from build123d import *

# Parameters (mm, degrees)
F0_W     = 100.4
F0_H     = 100.4
F0_W_2   = 87.7
F0_H_2   = 87.7
F1_DEPTH = 6.35
F2_DEPTH = 119.05


with BuildPart() as f1:
    # F0 (on Front) → F1 (new body)
    with BuildSketch(Plane.XZ):
        with Locations((0, 50.2)):
            Rectangle(F0_W, F0_H)
        with Locations((0, 50.2)):
            Rectangle(F0_W_2, F0_H_2, mode=Mode.SUBTRACT)
        with Locations((0, 50.2)):
            Rectangle(F0_W_2, F0_H_2)
    extrude(amount=F1_DEPTH)

    # F0 (on Front) → F2 (join)
    with BuildSketch(Plane.XZ):
        with Locations((0, 50.2)):
            Rectangle(F0_W, F0_H)
        with Locations((0, 50.2)):
            Rectangle(F0_W_2, F0_H_2, mode=Mode.SUBTRACT)
    extrude(amount=F2_DEPTH)


solid = f1.part
Verification items for the finished model (mm, model axes). A direction names the side the tool comes from. Coordinates: 2 decimals unless noted, no trailing zeros. Order: outer loops, then holes, each group sorted by start corner. A loop starts at its lowest first (then second) coordinate and runs counter-clockwise, first axis right, second up.
1. Sectioned sample at B-B, the plane z = 44. Record the cut outline in (x, y).
Results found:
outline: (-50.2, -119.05) - (-43.85, -119.05) - (-43.85, -6.35) - (43.85, -6.35) - (43.85, -119.05) - (50.2, -119.05) - (50.2, 0) - (-50.2, 0) - close
2. Sectioned sample at C-C, the plane x = 0. Record the cut outline in (y, z), and give its area (3 significant figures).
Results found:
outline: (-119.05, 0) - (0, 0) - (0, 100.4) - (-119.05, 100.4) - (-119.05, 94.05) - (-6.35, 94.05) - (-6.35, 6.35) - (-119.05, 6.35) - close
area: 2,070 mm2
3. Set-up check for faces 5 (the face through (-1, -119.05, 96)), 6 (the face through (-1, -62, 94.05)): record each of +Z, -Z, +X, -X, +Y, -Y from which the full face is reachable in a straight line by a thin tool's end or side.
Results found:
face 5: +Z, -Z, +X, -X, -Y
face 6: -Y
4. Release check for a two-part mould opening along X. For faces 1 (the face through (-50.2, -59, 49)), 2 (the face through (50.2, -59, 49)), 3 (the face through (43.85, -62, 50)), 4 (the face through (-1, -59, 100.4)) record: +X half, -X half, draft (parallel to the pull), parting line (faces both ways), or undercut.
Results found:
face 1: -X half
face 2: +X half
face 3: undercut
face 4: draft
5. Scan lines: line 1 (Z direction, x = -36.5, y = -44); line 2 (X direction, y = -17, z = 49); line 3 (Y direction, x = 40, z = 83.5). Record each from-to range of solid material in increasing order.
Results found:
line 1: z = 0 to 6.35, 94.05 to 100.4
line 2: x = -50.2 to -43.85, 43.85 to 50.2
line 3: y = -6.35 to 0
6. Sectioned sample at A-A, the plane y = -42.5. Record the cut outline in (x, z).
Results found:
outline: (-50.2, 0) - (50.2, 0) - (50.2, 100.4) - (-50.2, 100.4) - close; hole (-43.85, 6.35) - (43.85, 6.35) - (43.85, 94.05) - (-43.85, 94.05) - close
